For this review, take the finished solid that the model builds, in its own axes (mm). Face numbers are marked on the shaded views. A direction names the side the tool comes from. Give positions to 0.01 mm unless a question says otherwise; leave off trailing zeros. Order: outer loops, then holes, each group sorted by start corner. A loop starts at its lowest first (then second) coordinate and runs counter-clockwise, first axis right, second up. Notation, with made-up numbers: (-22, 46.25) - (0, 46.25) arc R22 ccw to (0, 63.25) - close; hole circle Ø8 at (-34, 0). An arc over 180 degrees is marked (long way). One line per item, written item: value.
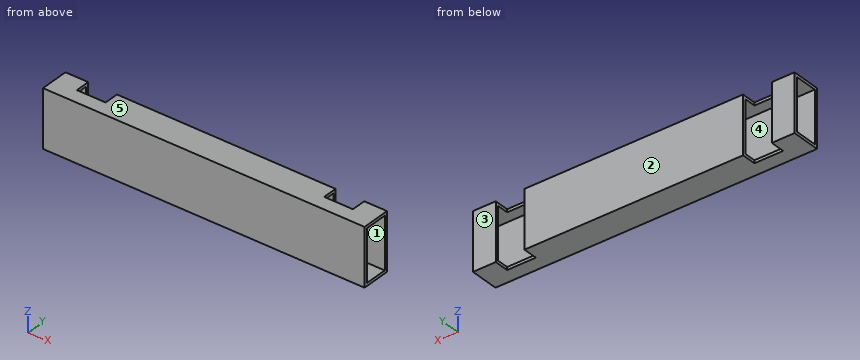
```python
from build123d import *

# Parameters (mm, degrees)
F0_W     = 355.6
F0_H     = 63.5
F1_DEPTH = 31.75
F2_W     = 31.75
F2_H     = 16.01724
F3_DEPTH = 63.501
F4_W     = 25.4
F4_H     = 57.15
F5_DEPTH = 355.601


with BuildPart() as f1:
    # F0 (on Front) → F1 (new body)
    with BuildSketch(Plane.XZ):
        with Locations((177.8, 31.75)):
            Rectangle(F0_W, F0_H)
    extrude(amount=F1_DEPTH)

    # F2 (on face) → F3 (cut, through all)
    with BuildSketch(Plane.XY.offset(63.5)):
        with Locations((41.06418, -8.00862)):
            Rectangle(F2_W, F2_H)
        with Locations((314.53582, -8.00862)):
            Rectangle(F2_W, F2_H)
    extrude(amount=-F3_DEPTH, mode=Mode.SUBTRACT)

    # F4 (on face) → F5 (cut, through all)
    with BuildSketch(Plane(origin=(0, 0, 0), x_dir=(0, -1, 0), z_dir=(-1, 0, 0))):
        with Locations((15.875, 31.75)):
            Rectangle(F4_W, F4_H)
    extrude(amount=-F5_DEPTH, mode=Mode.SUBTRACT)


solid = f1.part
```
(1) Draft analysis for pull direction Z (two halves, no side actions). For the marked faces 3, 4 and 5, state which applies: pulls with the +Z half, pulls with the -Z half, needs draft (parallel to the pull), parting line crosses it, or undercut.
Answers below:
face 3: needs draft
face 4: undercut
face 5: pulls with the +Z half
(2) Machinability: for the marked faces 1 and 2, which of the approach directions +Z, -Z, +X, -X, +Y, -Y give a long, thin tool a straight path to every point of the face, cutting with its end or side? Answer none if there is none.
Answers below:
face 1: +X, -X
face 2: +Z, -Z, +X, -X, +Y
(3) Take a section at C-C (x = 89). Write out the cut boundary in (y, z) (3 decimals).
Answers below:
outline: (-31.75, 0) - (0, 0) - (0, 63.5) - (-31.75, 63.5) - close; hole (-28.575, 3.175) - (-3.175, 3.175) - (-3.175, 60.325) - (-28.575, 60.325) - close
(4) Take a section at A-A (y = -25). Write out the cut boundary in (x, z) (3 decimals), then the cut area to 3 significant figures.
Answers below:
outline: (0, 0) - (355.6, 0) - (355.6, 3.175) - (0, 3.175) - close; (0, 60.325) - (355.6, 60.325) - (355.6, 63.5) - (0, 63.5) - close
area: 2,260 mm^2
(5) For P1, Ø13, axis at y = -11.5, z = 38.5, coming from the -X side; P2, Ø3.5, axis at x = 310, z = 2, coming from the +Y side, all flat-tipped, find the tip position at first contact; note any pin that passes through.
Answers below:
P1: passes through
P2: stops at y = -16.02
(6) Wall thickness on line 1 (X direction, y = -3, z = 31); line 2 (Z direction, x = 178.5, y = -23) (3 decimals); line 3 (Y direction, x = 230.5, z = 46.5) (3 decimals): over which ranges is each line inside the solid? List them lowest first. Write a range as from..to.
Answers below:
line 1: x = 0..25.19, 56.94..298.66, 330.41..355.6
line 2: z = 0..3.175, 60.325..63.5
line 3: y = -31.75..-28.575, -3.175..0
(7) Take a section at D-D (y = -8). Write out the cut boundary in (x, z) (3 decimals), then the cut area to 3 significant figures.
Answers below:
outline: (0, 0) - (25.189, 0) - (25.189, 3.175) - (0, 3.175) - close; (0, 60.325) - (25.189, 60.325) - (25.189, 63.5) - (0, 63.5) - close; (56.939, 0) - (298.661, 0) - (298.661, 3.175) - (56.939, 3.175) - close; (56.939, 60.325) - (298.661, 60.325) - (298.661, 63.5) - (56.939, 63.5) - close; (330.411, 0) - (355.6, 0) - (355.6, 3.175) - (330.411, 3.175) - close; (330.411, 60.325) - (355.6, 60.325) - (355.6, 63.5) - (330.411, 63.5) - close
area: 1,850 mm^2
(8) Take a section at B-B (z = 8). Write out the cut boundary in (x, y) (3 decimals).
Answers below:
outline: (0, -31.75) - (355.6, -31.75) - (355.6, -28.575) - (0, -28.575) - close; (0, -3.175) - (25.189, -3.175) - (25.189, 0) - (0, 0) - close; (56.939, -3.175) - (298.661, -3.175) - (298.661, 0) - (56.939, 0) - close; (330.411, -3.175) - (355.6, -3.175) - (355.6, 0) - (330.411, 0) - close
